Could you check a few things on this drawing? It's one solid part, dimensions in mm from its lowest x, y, z. A direction names the side the tool comes from. Give positions to 0.01 mm unless a question says otherwise; leave off trailing zeros. Order: outer loops, then holes, each group sorted by start corner. A loop starts at its lowest first (then second) coordinate and runs counter-clockwise, first axis right, second up.
Item 1: I want a section at C-C, the plane x = 16. Write out the boundary of the cut face in (y, z), then the cut area to 3 significant figures.
Item 2: I want a section at D-D, the plane y = 22. Write out the boundary of the cut face in (x, z), then the cut area to 3 significant figures.
Item 3: I'm going to push flat-ended pins straight in: pin 1 Ø5 at (x, y) = (13, 16.5) entering from -Z; pin 2 Ø5 at (y, z) = (19.5, 5.5) entering from -X; pin 3 Ø4 at (x, y) = (14.5, 27) entering from +Z; pin 4 Ø2 at (x, z) = (30, 8.5) entering from -Y. Where does each tip first touch, or does it pass through?
Item 4: If I drill on line 1 along Z through (x, y) = (10, 13) (1 decimal); line 2 along X through (y, z) = (23, 28.5); line 3 along X through (y, z) = (31, 29), over which ranges is the centre line in solid material (lowest first)?
Item 5: Which directions (+Z, -Z, +X, -X, +Y, -Y) give clear straight access to the entire face, cutting with the end or side of a thin tool? Please do the marked faces 1, 2 and 3.
Item 6: I want a section at B-B, the plane y = 39.5. Write out the boundary of the cut face in (x, z).
Item 7: I want a section at A-A, the plane z = 9. Write out the boundary of the cut face in (x, y).
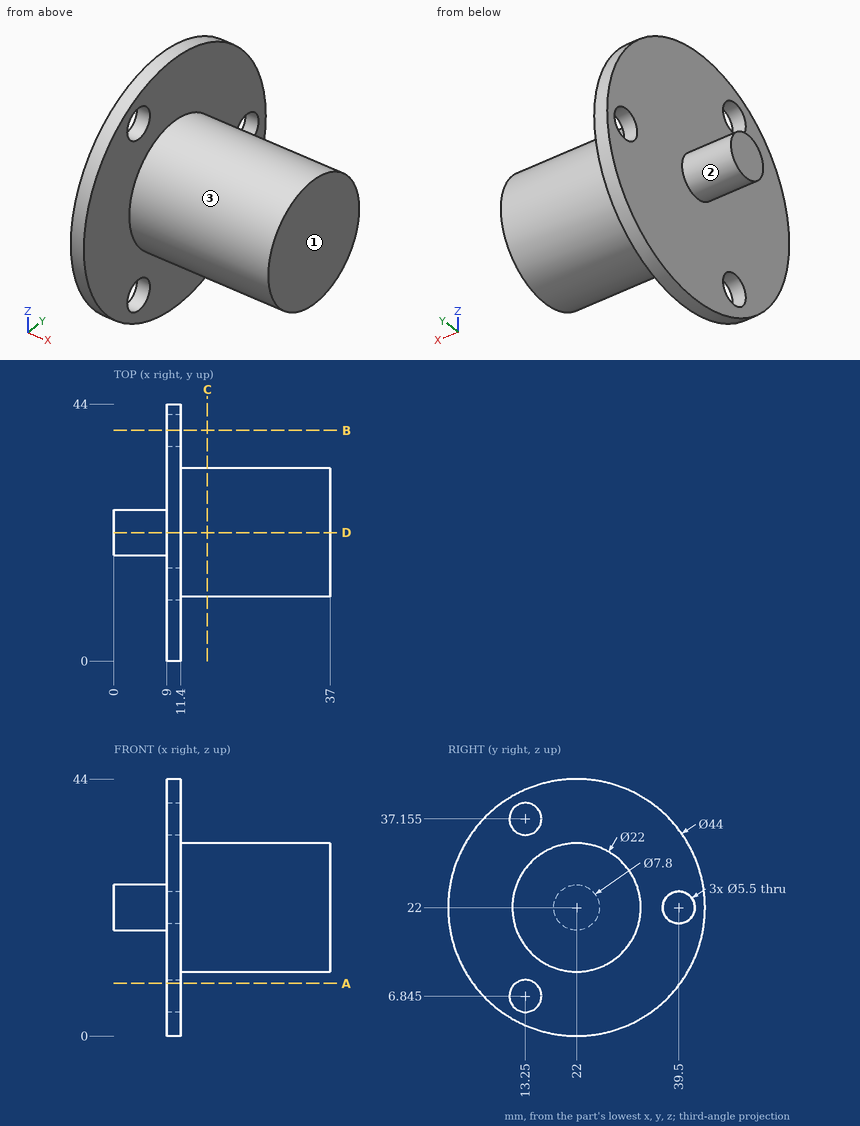
Results list:
1. outline: circle Ø22 at (22, 22)
1. area: 380 mm2
2. outline: (0, 18.1) - (9, 18.1) - (9, 0) - (11.4, 0) - (11.4, 11) - (37, 11) - (37, 33) - (11.4, 33) - (11.4, 44) - (9, 44) - (9, 25.9) - (0, 25.9) - close
2. area: 739 mm2
3. pin 1: stops at z = 0.29
3. pin 2: stops at x = 9
3. pin 3: stops at z = 32.58
3. pin 4: passes through
4. line 1: z = 1.9 to 4.1, 9.6 to 34.4, 39.9 to 42.1
4. line 2: x = 9 to 37
4. line 3: x = 9 to 11.4
5. face 1: +Z, -Z, +X, +Y, -Y
5. face 2: -X
5. face 3: +X
6. outline: (9, 8.67) - (11.4, 8.67) - (11.4, 19.25) - (9, 19.25) - close; (9, 24.75) - (11.4, 24.75) - (11.4, 35.33) - (9, 35.33) - close
7. outline: (9, 4.25) - (11.4, 4.25) - (11.4, 11.54) - (9, 11.54) - close; (9, 14.96) - (11.4, 14.96) - (11.4, 39.75) - (9, 39.75) - close
